Source: CAD feature listing. Evaluate the final solid. Frame: model axes, mm. A direction names the side the tool comes from. Round coordinates to 2 decimals unless told otherwise and drop trailing zeros. Write each loop counter-clockwise with the first axis right and the second up, starting at its lowest first coordinate (ties: lowest second). Pieces come first, ordered by that corner, then holes. Notation, with made-up numbers: (-5, 69) -> (52, 69) arc R27 cw to (52, 91) -> close; hole circle Ø1 at (64.5, 34.5). An arc over 180 degrees is marked (long way). Put each result on its own line as item: value.
```python
from build123d import *

# Parameters (mm, degrees)
F1_DEPTH = 20
F3_DEPTH = 3
F4_R     = 5
F5_DEPTH = 3


with BuildPart() as f1:
    # F0 (on Top) → F1 (new body)
    with BuildSketch(Plane.XY):
        Polygon((0.95669, 33), (0.95669, 0), (0.95669, -33), (17.058177, -33), (13.95669, -30), (13.95669, -31), (2.95669, -31), (2.95669, 0), (2.95669, 31), (13.95669, 31), (13.95669, 30), (17.058177, 33), align=None)
    extrude(amount=F1_DEPTH)

    # F2 (on face) → F3 (join)
    with BuildSketch(Plane(origin=(0.95669, 0, 0), x_dir=(0, -1, 0), z_dir=(-1, 0, 0))):
        with BuildLine():
            ThreePointArc((2.5, 10), (1.767767, 11.767767), (0, 12.5))
            Line((0, 12.5), (0, 10))
            Line((0, 10), (2.5, 10))
        make_face()
        with BuildLine():
            Line((0, 10), (0, 12.5))
            ThreePointArc((0, 12.5), (-1.767767, 11.767767), (-2.5, 10))
            Line((-2.5, 10), (0, 10))
        make_face()
        with BuildLine():
            Line((2.5, 10), (0, 10))
            Line((0, 10), (0, 7.5))
            ThreePointArc((0, 7.5), (1.767767, 8.232233), (2.5, 10))
        make_face()
        with BuildLine():
            Line((0, 7.5), (0, 10))
            Line((0, 10), (-2.5, 10))
            ThreePointArc((-2.5, 10), (-1.767767, 8.232233), (0, 7.5))
        make_face()
    extrude(amount=F3_DEPTH)

    # F4 (on face) → F5 (join)
    with BuildSketch(Plane(origin=(-2.04331, 0, 0), x_dir=(0, -1, 0), z_dir=(-1, 0, 0))):
        with Locations((0, 10)):
            Circle(F4_R)
    extrude(amount=F5_DEPTH)


solid = f1.part
```
Q1. Cut plane C-C on z = 17. Output: boundary loops of the cut face in (x, y), and give its area (3 significant figures).
Ans:
outline: (0.96, -33) -> (17.06, -33) -> (13.96, -30) -> (13.96, -31) -> (2.96, -31) -> (2.96, 31) -> (13.96, 31) -> (13.96, 30) -> (17.06, 33) -> (0.96, 33) -> close
area: 185 mm^2
Q2. Draft query along X for faces 6 (the flat face through (-2.043, -2, 8)), 7 (the flat face through (15.486, 31.479, 9.86)), 8 (the flat face through (8, 31, 10)), 9 (the flat face through (2, 0, 20)). Return one class per face: +X half, -X half, draft (parallel to the pull), parting line (faces both ways), or undercut.
Ans:
face 6: undercut
face 7: +X half
face 8: undercut
face 9: draft
Q3. Reachability of faces 1 (the flat face through (2, 0, 0)), 2 (the flat face through (9, 33, 10)), 3 (the flat face through (9, -31, 10)), 4 (the flat face through (15.53, -31.52, 9.86)), 5 (the cylindrical face through (-3.522, 0.651, 14.957)) from +Z, -Z, +X, -X, +Y, -Y: full face, straight path, thin tool, end or side. Return the list, or none.
Ans:
face 1: -Z, +X, -X, +Y, -Y
face 2: +Z, -Z, +X, -X, +Y
face 3: +Z, -Z
face 4: +Z, -Z, +X
face 5: -X
Q4. Material intervals for line 1 (Y direction, x = 5, z = 7); line 2 (X direction, y = -1, z = 13.25); line 3 (X direction, y = 7, z = 4), sorted ascending. Write a range as [from, to].
Ans:
line 1: y = [-33, -31], [31, 33]
line 2: x = [-5.04, -2.04], [0.96, 2.96]
line 3: x = [0.96, 2.96]
Q5. Cut plane B-B on x = 7.5. Output: boundary loops of the cut face in (y, z).
Ans:
outline: (-33, 0) -> (-31, 0) -> (-31, 20) -> (-33, 20) -> close; (31, 0) -> (33, 0) -> (33, 20) -> (31, 20) -> close
Q6. Cut plane A-A on z = 6. Output: boundary loops of the cut face in (x, y).
Ans:
outline: (-5.04, -3) -> (-2.04, -3) -> (-2.04, 3) -> (-5.04, 3) -> close; (0.96, -33) -> (17.06, -33) -> (13.96, -30) -> (13.96, -31) -> (2.96, -31) -> (2.96, 31) -> (13.96, 31) -> (13.96, 30) -> (17.06, 33) -> (0.96, 33) -> close
Q7. Pin query (flat end, axial travel): pin 1 (5 mm diameter, centred on y = -2.5, z = 10, fed in from +X); pin 2 (4 mm diameter, centred on y = 24.5, z = 10.5, fed in from -X). Return the tip coordinate at first contact, or that it passes through.
Ans:
pin 1: stops at x = 2.96
pin 2: stops at x = 0.96
Q8. Cut plane D-D on y = -8.5. Output: boundary loops of the cut face in (x, z), and give its area (3 significant figures).
Ans:
outline: (0.96, 0) -> (2.96, 0) -> (2.96, 20) -> (0.96, 20) -> close
area: 40.0 mm^2
